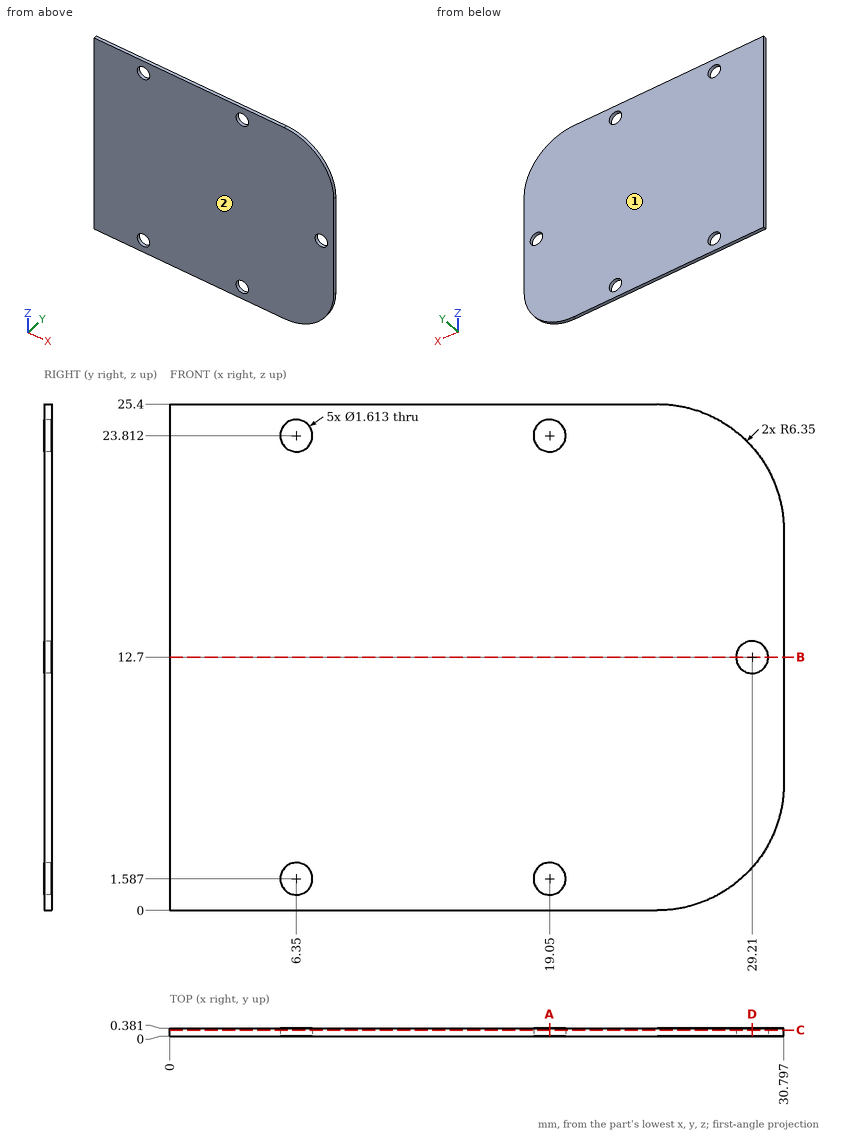
Part print with two shaded views. Sizes in mm from the minimum x, y, z corner. Round coordinates to 2 decimals unless told otherwise and drop trailing zeros. Order: outer loops, then holes, each group sorted by start corner. A loop starts at its lowest first (then second) coordinate and runs counter-clockwise, first axis right, second up. Notation, with made-up numbers: M -18,-6 L 22,-6 A38 cw 22,32 Z; hole C 75.25,15.5 d8. An arc over 180 degrees is marked long. Use CSV: the item, a comma, the result in double quotes.
Item 1: Saw through at B-B (z = 12.7). List the corners of the cut face in (x, y).
Worked answers:
outline,"M 0,0 L 28.4,0 L 28.4,0.38 L 0,0.38 Z; M 30.02,0 L 30.8,0 L 30.8,0.38 L 30.02,0.38 Z"
Item 2: Saw through at D-D (x = 29.21). List the corners of the cut face in (y, z).
Worked answers:
outline,"M 0,2.15 L 0.38,2.15 L 0.38,11.89 L 0,11.89 Z; M 0,13.51 L 0.38,13.51 L 0.38,23.25 L 0,23.25 Z"
Item 3: Saw through at A-A (x = 19.05). List the corners of the cut face in (y, z).
Worked answers:
outline,"M 0,0 L 0.38,0 L 0.38,0.78 L 0,0.78 Z; M 0,2.39 L 0.38,2.39 L 0.38,23.01 L 0,23.01 Z; M 0,24.62 L 0.38,24.62 L 0.38,25.4 L 0,25.4 Z"
Item 4: Saw through at C-C (y = 0.3). List the corners of the cut face in (x, z), plus the area to 3 significant figures.
Worked answers:
outline,"M 0,0 L 24.45,0 A6.35 ccw 30.8,6.35 L 30.8,19.05 A6.35 ccw 24.45,25.4 L 0,25.4 Z; hole C 6.35,1.59 d1.61; hole C 6.35,23.81 d1.61; hole C 19.05,1.59 d1.61; hole C 19.05,23.81 d1.61; hole C 29.21,12.7 d1.61"
area,"755 mm²"
Item 5: Pin check, flat tips, straight feed: pin 1 (1.3 mm diameter, centred on x = 29.21, z = 12.7, fed in from +Y); pin 2 (2.5 mm diameter, centred on x = 19.05, z = 1.59, fed in from +Y). Stop position of each tip, or through.
Worked answers:
pin 1,"through"
pin 2,"y = 0.38"
Item 6: Probe probe 1 along Z at (x, y) = (19.05, 0.25); probe 2 along Z at (x, y) = (6, 0.2) (1 decimal); probe 3 along X at (y, z) = (0.1, 23.25) (1 decimal). List the from-to ranges inside material, lowest first.
Worked answers:
probe 1,"0 to 0.78, 2.39 to 23.01, 24.62 to 25.4"
probe 2,"0 to 0.9, 2.3 to 23.1, 24.5 to 25.4"
probe 3,"0 to 5.8, 6.9 to 18.5, 19.6 to 29.2"
Item 7: Pull direction Y, two halves, no side cores. Call the marked faces 1 and 2: released by +Y, released by -Y, zero draft, split by the parting line, or undercut.
Worked answers:
face 1,"released by +Y"
face 2,"released by -Y"
